Can you work these out from the model? Positions are in its coordinate system, mm. A direction names the side the tool comes from. Give positions to 0.01 mm unless a question says otherwise; leave off trailing zeros. Write each loop counter-clockwise with the first axis right and the second up, starting at its lowest first coordinate (ties: lowest second). Pieces come first, ordered by that corner, then holes. Notation, with made-up numbers: (74, 78) -> (84, 78) arc R22 ccw to (84, 90) -> close; hole circle Ø3 at (75, 42). An arc over 180 degrees is marked (long way). One line per item, written item: value.
from build123d import *

# Parameters (mm, degrees)
F0_W      = 620
F0_H      = 620
F1_DEPTH  = 3
F2_W      = 620
F2_H      = 620
F2_W_2    = 616
F2_H_2    = 616
F3_DEPTH  = 25
F4_DEPTH  = 25
F5_W      = 150
F5_H      = 20
F6_DEPTH  = 60
F7_W      = 140
F7_H      = 55
F8_DEPTH  = 25
F9_W      = 20
F9_H      = 30
F10_DEPTH = 40
F11_R     = 6
F12_DEPTH = 540.001


with BuildPart() as f1:
    # F0 (on Top) → F1 (new body)
    with BuildSketch(Plane.XY):
        Rectangle(F0_W, F0_H)
    extrude(amount=F1_DEPTH)

    # F2 (on face) → F3 (join)
    with BuildSketch(Plane(origin=(0, 0, 0), x_dir=(1, 0, 0), z_dir=(0, 0, -1))):
        Rectangle(F2_W, F2_H)
        Rectangle(F2_W_2, F2_H_2, mode=Mode.SUBTRACT)
    extrude(amount=F3_DEPTH)

    # F4 (add): a face of the model
    f4_faces = [f1.faces().sort_by_distance(p)[0] for p in [
        (0, 0, 3),
    ]]
    extrude(f4_faces, amount=F4_DEPTH)

    # F5 (on face) → F6 (join)
    with BuildSketch(Plane.XZ.offset(310)):
        with Locations((175, 18)):
            Rectangle(F5_W, F5_H)
    extrude(amount=F6_DEPTH)

    # F7 (on face) → F8 (cut)
    with BuildSketch(Plane.XY.offset(28)):
        with Locations((175, -337.5)):
            Rectangle(F7_W, F7_H)
    extrude(amount=-F8_DEPTH, mode=Mode.SUBTRACT)

    # F9 (on face) → F10 (join)
    with BuildSketch(Plane(origin=(0, 310, 0), x_dir=(-1, 0, 0), z_dir=(0, 1, 0))):
        with Locations((220, 6)):
            Rectangle(F9_W, F9_H)
        with Locations((-220, 6)):
            Rectangle(F9_W, F9_H)
    extrude(amount=F10_DEPTH)

    # F11 (on face) → F12 (cut, through all)
    with BuildSketch(Plane.YZ.offset(230)):
        with Locations((338, 6)):
            Circle(F11_R)
    extrude(amount=-F12_DEPTH, mode=Mode.SUBTRACT)


solid = f1.part
1) If we section it at A-A (y = 65.5): Write out the boundary of the cut face in (x, z).
Answer list:
outline: (-310, -25) -> (-308, -25) -> (-308, 0) -> (308, 0) -> (308, -25) -> (310, -25) -> (310, 28) -> (-310, 28) -> close
2) I need wall thicknesses on L1, parallel to X at y = -47.5, z = -22; L2, parallel to Z at x = -218, y = 338. Which ranges of each line are inside material? Lowest first, please.
Answer list:
L1: x = -310 to -308, 308 to 310
L2: z = -9 to 0, 12 to 21
3) We'd pull the mould along X, two halves only. Please class faces 6 (the face through (250, -340, 18)), 7 (the face through (-4, 310, 1)), 8 (the face through (220, 330, -9)): released by +X, released by -X, zero draft, split by the parting line, or undercut.
Answer list:
face 6: released by +X
face 7: undercut
face 8: zero draft
4) For faces 1 (the face through (308, 4, -12)), 2 (the face through (-220, 330, -9)), 3 (the face through (220, 330, 21)), 4 (the face through (-230, 330, 6)), 5 (the face through (174, -365, 18)), which set-ups out of +Z, -Z, +X, -X, +Y, -Y let a thin tool reach every point of the face, with its end or its side?
Answer list:
face 1: -Z
face 2: -Z, +X, -X, +Y
face 3: +Z, +X, -X, +Y
face 4: +Z, -Z, -X, +Y
face 5: +Z, -Z
5) Will these pins go through, and if not, where does the flat tip stop? pin 1 (12 mm diameter, centred on x = -7, y = 269, fed in from -Z); pin 2 (4 mm diameter, centred on x = -168.5, z = -2.5, fed in from +Y); pin 3 (10 mm diameter, centred on x = -220, y = 328.5, fed in from -Z); pin 4 (9.5 mm diameter, centred on y = 338, z = 6, fed in from -X).
Answer list:
pin 1: stops at z = 0
pin 2: stops at y = 310
pin 3: stops at z = -9
pin 4: passes through
